The figure shows three views and two pictorial views of one solid part (mm, origin at its lowest corner). Answer the questions. Coordinates: 2 decimals unless noted, no trailing zeros. Order: outer loops, then holes, each group sorted by start corner. A loop starts at its lowest first (then second) coordinate and runs counter-clockwise, first axis right, second up. Notation, with made-up numbers: M 48,59 L 89,59 A24 ccw 89,84 Z; hole C 12,-21 d8. An arc over 180 degrees is marked long. Use a Markdown table: item, result.
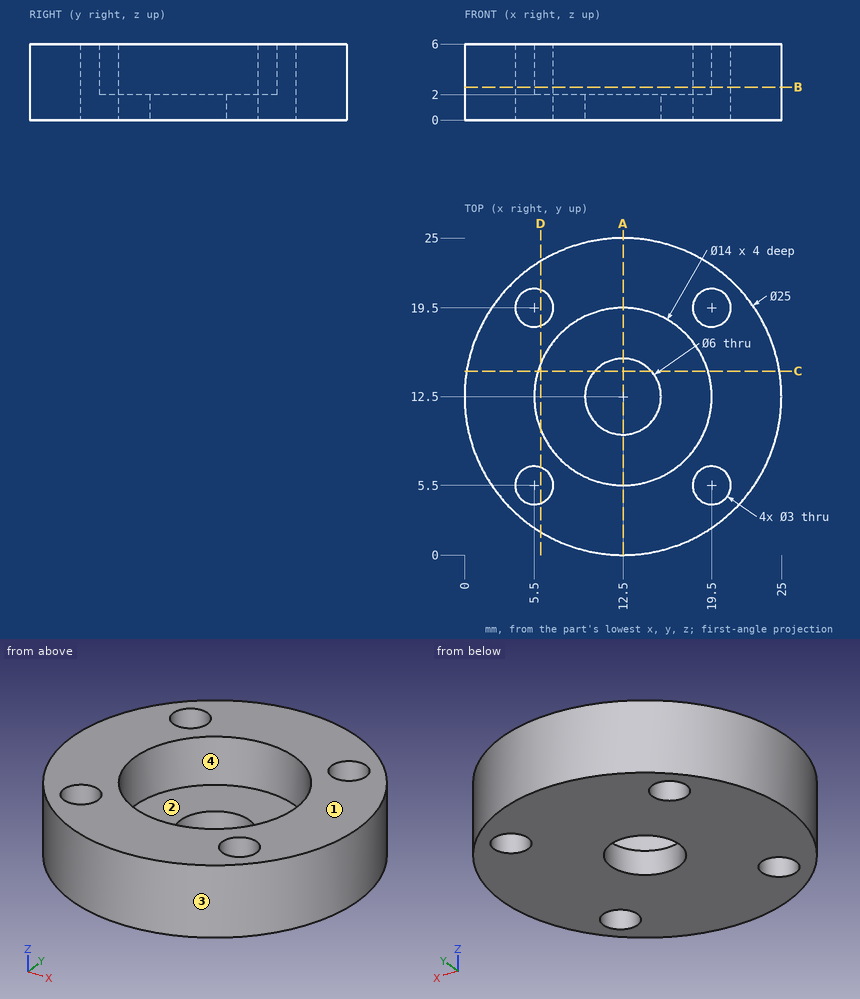
1. Section A-A on x = 12.5 is taken. Determine the outline of the cut face in (y, z).
Answers below:
| item | result |
|---|---|
| outline | M 0,0 L 9.5,0 L 9.5,2 L 5.5,2 L 5.5,6 L 0,6 Z; M 15.5,0 L 25,0 L 25,6 L 19.5,6 L 19.5,2 L 15.5,2 Z |
2. Section C-C on y = 14.5 is taken. Determine the outline of the cut face in (x, z), then the cut area to 3 significant figures.
Answers below:
| item | result |
|---|---|
| outline | M 0.16,0 L 10.26,0 L 10.26,2 L 5.79,2 L 5.79,6 L 0.16,6 Z; M 14.74,0 L 24.84,0 L 24.84,6 L 19.21,6 L 19.21,2 L 14.74,2 Z |
| area | 85.5 mm² |
3. Flat-ended cylindrical pins translate along their axes: P1, Ø2, axis at x = 15, z = 4, coming from the -Y side; P2, Ø1.5, axis at y = 21.5, z = 2, coming from the -X side; P3, Ø7, axis at x = 11.5, y = 15, coming from the +Z side. Find the tip coordinate at first contact, or state that the pin passes through.
Answers below:
| item | result |
|---|---|
| P1 | y = 0.09 |
| P2 | x = 3.11 |
| P3 | z = 2 |
4. Section B-B on z = 2.6 is taken. Determine the outline of the cut face in (x, y), then the cut area to 3 significant figures.
Answers below:
| item | result |
|---|---|
| outline | C 12.5,12.5 d25; hole C 5.5,5.5 d3; hole C 5.5,19.5 d3; hole C 12.5,12.5 d14; hole C 19.5,5.5 d3; hole C 19.5,19.5 d3 |
| area | 309 mm² |
5. Section D-D on x = 6 is taken. Determine the outline of the cut face in (y, z).
Answers below:
| item | result |
|---|---|
| outline | M 1.82,0 L 4.09,0 L 4.09,6 L 1.82,6 Z; M 6.91,0 L 18.09,0 L 18.09,6 L 15.1,6 L 15.1,2 L 9.9,2 L 9.9,6 L 6.91,6 Z; M 20.91,0 L 23.18,0 L 23.18,6 L 20.91,6 Z |
6. Find the intervals of material crossed by probe 1 along Y at (x, z) = (12.5, 4.8); probe 2 along Y at (x, z) = (5.5, 1.9); probe 3 along Z at (x, y) = (7, 8.5), in increasing order.
Answers below:
| item | result |
|---|---|
| probe 1 | 0 to 5.5, 19.5 to 25 |
| probe 2 | 2.14 to 4, 7 to 18, 21 to 22.86 |
| probe 3 | 0 to 2 |
7. For a pull along Y with two mould halves and no side action, classify the marked faces 1, 2, 3 and 4 as +Y half, -Y half, draft (parallel to the pull), parting line (faces both ways), or undercut.
Answers below:
| item | result |
|---|---|
| face 1 | draft |
| face 2 | undercut |
| face 3 | parting line |
| face 4 | undercut |
